Verification items for the finished model (mm, model axes). Face numbers are marked on the shaded views. A direction names the side the tool comes from. Give positions to 0.01 mm unless a question says otherwise; leave off trailing zeros. Order: outer loops, then holes, each group sorted by start corner. A loop starts at its lowest first (then second) coordinate and runs counter-clockwise, first axis right, second up.
(1) Sectioned sample at C-C on y = 2.5. Record the cut outline in (x, z).
(2) Scan lines: L1, parallel to Z at x = 36, y = -1; L2, parallel to X at y = -0.5, z = 24.5; L3, parallel to X at y = 8.5, z = 38. Record each from-to range of solid material in increasing order.
(3) Mould release check, pull along Z, two halves, no side actions. Record for the marked faces 4, 5, 6 and 7: pulls with the +Z half, pulls with the -Z half, needs draft (parallel to the pull), parting line crosses it, or undercut.
(4) Access from +Z, -Z, +X, -X, +Y, -Y to the whole of each face (thin tool, end or side, straight path). Record for the marked faces 1, 2 and 3.
(5) Sectioned sample at B-B on x = 37. Record the cut outline in (y, z).
(6) Sectioned sample at D-D on x = 24. Record the cut outline in (y, z), plus the area to 3 significant figures.
(7) Gauge pin test, flat ends, axial feed: pin 1 (3 mm diameter, centred on y = 0, z = 18, fed in from -X); pin 2 (1.6 mm diameter, centred on x = 20, y = 4, fed in from +Z); pin 3 (5 mm diameter, centred on y = 5, z = 18, fed in from +X). Record the tip position at first contact, or that the pin passes through.
(8) Sectioned sample at A-A on z = 30. Record the cut outline in (x, y), plus the area to 3 significant figures.
```python
from build123d import *

# Parameters (mm, degrees)
F1_DEPTH = 12.5


with BuildPart() as f1:
    # F0 (on Front) → F1 (new body, symmetric)
    with BuildSketch(Plane.XZ):
        Polygon((0, 15), (0, 0), (10, 0), (19, 9), (19, 11), (21, 11), (21, 9), (30, 0), (40, 0), (40, 15), (34, 15), (34, 25), (40, 25), (40, 40), (35, 40), (21, 26), (21, 24), (19, 24), (19, 26), (5, 40), (0, 40), (0, 25), (6, 25), (6, 15), align=None)
    extrude(amount=F1_DEPTH, both=True)


solid = f1.part
```
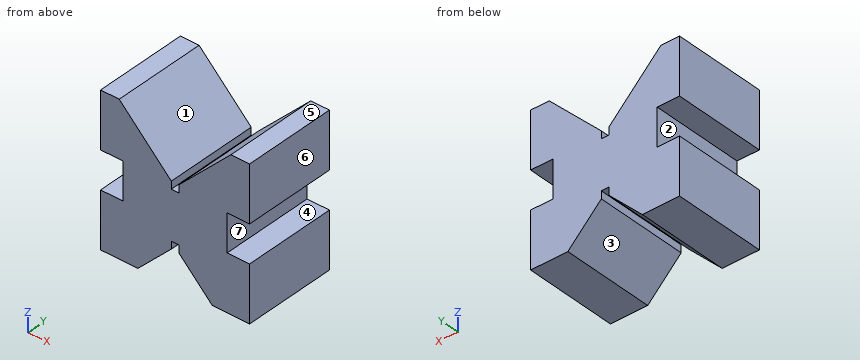
Ans:
1. outline: (0, 0) - (10, 0) - (19, 9) - (19, 11) - (21, 11) - (21, 9) - (30, 0) - (40, 0) - (40, 15) - (34, 15) - (34, 25) - (40, 25) - (40, 40) - (35, 40) - (21, 26) - (21, 24) - (19, 24) - (19, 26) - (5, 40) - (0, 40) - (0, 25) - (6, 25) - (6, 15) - (0, 15) - close
2. L1: z = 0 to 15, 25 to 40
2. L2: x = 6 to 19, 21 to 34
2. L3: x = 0 to 7, 33 to 40
3. face 4: undercut
3. face 5: pulls with the +Z half
3. face 6: needs draft
3. face 7: undercut
4. face 1: +Z, +Y, -Y
4. face 2: -X, +Y, -Y
4. face 3: -Z, +Y, -Y
5. outline: (-12.5, 0) - (12.5, 0) - (12.5, 15) - (-12.5, 15) - close; (-12.5, 25) - (12.5, 25) - (12.5, 40) - (-12.5, 40) - close
6. outline: (-12.5, 6) - (12.5, 6) - (12.5, 29) - (-12.5, 29) - close
6. area: 575 mm2
7. pin 1: stops at x = 6
7. pin 2: stops at z = 24
7. pin 3: stops at x = 34
8. outline: (0, -12.5) - (15, -12.5) - (15, 12.5) - (0, 12.5) - close; (25, -12.5) - (40, -12.5) - (40, 12.5) - (25, 12.5) - close
8. area: 750 mm2
